from build123d import *

# Parameters (mm, degrees)
SZKIC2_R                    = 23.25
DODANIE_WYCI_GNI_CIE2_DEPTH = 40


with BuildPart() as part:
    # Szkic2 → Dodanie-wyciągnięcie2 (new body)
    with BuildSketch(Plane.XY):
        with BuildLine():
            Line((0, 0), (0, 54.688934957))
            Line((0, 54.688934957), (87.453362302, 248.067468892))
            ThreePointArc((87.453362302, 248.067468892), (87.993040755, 268.91551183), (73.44838199, 283.861583171))
            ThreePointArc((73.44838199, 283.861583171), (65.201876961, 289.507605405), (59.808019866, 297.921208552))
            ThreePointArc((59.808019866, 297.921208552), (83.279468744, 351.232430567), (136.626207071, 327.841816741))
            ThreePointArc((136.626207071, 327.841816741), (144.956248443, 312.604323506), (156.856823864, 299.957304331))
            Line((156.856823864, 299.957304331), (322.684534721, 163.527324946))
            ThreePointArc((322.684534721, 163.527324946), (344.192875478, 160.854554943), (355.793873119, 179.162183827))
            Line((355.793873119, 179.162183827), (355.793873119, 281.253729426))
            ThreePointArc((355.793873119, 281.253729426), (351.366678921, 300.628861995), (338.963821807, 316.158348333))
            ThreePointArc((338.963821807, 316.158348333), (366.011924038, 392.109534411), (391.227480575, 315.530436679))
            ThreePointArc((391.227480575, 315.530436679), (378.213678028, 299.824941516), (373.550822068, 279.968471302))
            Line((373.550822068, 279.968471302), (373.550822068, 154.228140368))
            ThreePointArc((373.550822068, 154.228140368), (380.150790995, 124.795180873), (398.686800685, 100.998646686))
            Line((398.686800685, 100.998646686), (462, 48.909533035))
            Line((462, 48.909533035), (462, 0))
            Line((462, 0), (0, 0))
        make_face()
        with Locations((96.5, 314)):
            Circle(SZKIC2_R, mode=Mode.SUBTRACT)
        with Locations((365.5, 349.5)):
            Circle(SZKIC2_R, mode=Mode.SUBTRACT)
        with BuildLine():
            Line((38.140490442, 21.985652154), (405.231641072, 21.985652154))
            ThreePointArc((405.231641072, 21.985652154), (424.253349591, 35.373578819), (418.06991605, 57.797385924))
            Line((418.06991605, 57.797385924), (149.573518435, 278.695074266))
            ThreePointArc((149.573518435, 278.695074266), (136.029024136, 281.900539629), (125.203881252, 273.151561656))
            Line((125.203881252, 273.151561656), (20.983248041, 48.87798069))
            ThreePointArc((20.983248041, 48.87798069), (22.19081724, 30.72910257), (38.140490442, 21.985652154))
        make_face(mode=Mode.SUBTRACT)
    extrude(amount=DODANIE_WYCI_GNI_CIE2_DEPTH)


solid = part.part
Geometry: final body of the model. Coordinates: model frame, mm. A direction names the side the tool comes from. Round coordinates to 2 decimals unless told otherwise and drop trailing zeros. Loops run counter-clockwise (first coordinate to the right, second up) from the corner with the lowest first, then second, coordinate; pieces in that order, holes last.
Q1. Section D-D on x = 110. Return loops of the section in (y, z), plus the area to 3 significant figures.
Q2. Access query for faces 4 (the flat face through (219, 21.986, 20)), 5 (the cylindrical face through (144.813, 312.802, 19.72)), 6 (the cylindrical face through (379.97, 125.18, 19.72)). Directions: +Z, -Z, +X, -X, +Y, -Y. A direction counts if a zero-diameter tool reaches every point of the face in a straight line with its end or side. Return the directions, or none.
Q3. Section A-A on x = 298. Return loops of the section in (y, z), plus the area to 3 significant figures.
Q4. Pull-direction query (X, two-part tool) for faces 1 (the flat face through (249.2, 197, 40)), 2 (the flat face through (355.794, 229, 20)), 3 (the cylindrical face through (88.1, 268.64, 19.72)); classes: released by +X, released by -X, zero draft, split by the parting line, or undercut.
Q5. Material intervals for L1, parallel to Y at x = 365.5, z = 30; L2, parallel to X at y = 183, z = 27.5; L3, parallel to Y at x = 93, z = 5, sorted ascending.
Q6. Pin query (flat end, axial travel): P1, Ø1, axis at y = 323, z = 15.5, coming from the +X side; P2, Ø6, axis at y = 140, z = 29, coming from the +X side; P3, Ø12, axis at x = 131, z = 14.5, coming from the +Y side. Return the tip coordinate at first contact, or that it passes through.
Q7. Section B-B on y = 266.5. Return loops of the section in (x, z).
Q8. Section C-C on z = 33. Return loops of the section in (x, y).
Evaluation:
1. outline: (0, 0) - (21.99, 0) - (21.99, 40) - (0, 40) - close; (240.43, 0) - (295.07, 0) - (295.07, 40) - (240.43, 40) - close; (332.93, 0) - (352.33, 0) - (352.33, 40) - (332.93, 40) - close
1. area: 3,840 mm2
2. face 4: +Z, -Z
2. face 5: +Z, -Z, +Y
2. face 6: +Z, -Z, +X
3. outline: (0, 0) - (21.99, 0) - (21.99, 40) - (0, 40) - close; (156.58, 0) - (183.84, 0) - (183.84, 40) - (156.58, 40) - close
3. area: 1,970 mm2
4. face 1: zero draft
4. face 2: undercut
4. face 3: released by -X
5. L1: y = 0 to 21.99, 101.05 to 326.25, 372.75 to 392.11
5. L2: x = 58.03 to 83.31, 265.89 to 299.02, 355.79 to 373.55
5. L3: y = 0 to 21.99, 203.85 to 291.01, 336.99 to 353.71
6. P1: stops at x = 399.26
6. P2: stops at x = 375.74
6. P3: stops at y = 344.18
7. outline: (88.81, 0) - (122.11, 0) - (122.11, 40) - (88.81, 40) - close; (164.4, 0) - (197.52, 0) - (197.52, 40) - (164.4, 40) - close; (355.79, 0) - (373.55, 0) - (373.55, 40) - (355.79, 40) - close
8. outline: (0, 0) - (462, 0) - (462, 48.91) - (398.69, 101) arc R68.93 cw to (373.55, 154.23) - (373.55, 279.97) arc R44.61 cw to (391.23, 315.53) arc R42.61 ccw (long way) to (338.96, 316.16) arc R44.61 cw to (355.79, 281.25) - (355.79, 179.16) arc R20.25 cw to (322.68, 163.53) - (156.86, 299.96) arc R68.36 cw to (136.63, 327.84) arc R41.22 ccw to (59.81, 297.92) arc R25.13 ccw to (73.45, 283.86) arc R26.85 cw to (87.45, 248.07) - (0, 54.69) - close; hole (20.98, 48.88) arc R18.92 ccw to (38.14, 21.99) - (405.23, 21.99) arc R20.21 ccw to (418.07, 57.8) - (149.57, 278.7) arc R15.8 ccw to (125.2, 273.15) - close; hole circle Ø46.5 at (96.5, 314); hole circle Ø46.5 at (365.5, 349.5)
